Check sheet for the drawn part. Datum: minimum x, y, z corner. Units: mm. Give positions to 0.01 mm unless a question says otherwise; leave off trailing zeros. Order: outer loops, then holes, each group sorted by start corner. A loop starts at its lowest first (then second) coordinate and runs counter-clockwise, first axis right, second up.
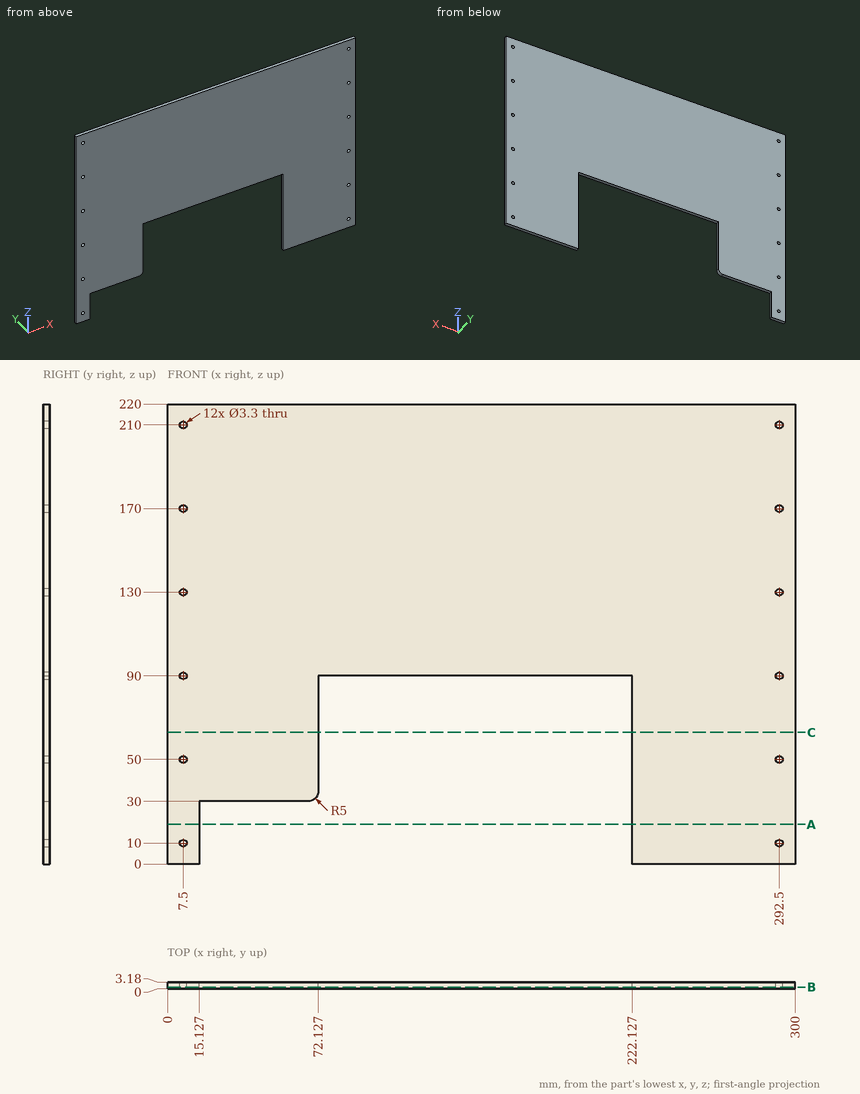
(1) Section check C-C, the plane z = 63. Enter the section's corners in (x, y).
Solved:
outline: (0, 0) - (72.13, 0) - (72.13, 3.18) - (0, 3.18) - close; (222.13, 0) - (300, 0) - (300, 3.18) - (222.13, 3.18) - close
(2) Go/stop test with flat-tipped pins: pin 1 (5.5 mm diameter, centred on x = 7.5, z = 10, fed in from +Y); pin 2 (3 mm diameter, centred on x = 292.5, z = 10, fed in from +Y); pin 3 (1 mm diameter, centred on x = 38.5, y = 1.5, fed in from -Z). Record where each tip stops, or that it passes through.
Solved:
pin 1: stops at y = 3.18
pin 2: passes through
pin 3: stops at z = 30
(3) Scan lines: line 1 (X direction, y = 0.95, z = 170); line 2 (X direction, y = 2.95, z = 44.5); line 3 (X direction, y = 1.8, z = 10). Record each from-to range of solid material in increasing order.
Solved:
line 1: x = 0 to 5.85, 9.15 to 290.85, 294.15 to 300
line 2: x = 0 to 72.13, 222.13 to 300
line 3: x = 0 to 5.85, 9.15 to 15.13, 222.13 to 290.85, 294.15 to 300
(4) Section check A-A, the plane z = 19. Enter the section's corners in (x, y).
Solved:
outline: (0, 0) - (15.13, 0) - (15.13, 3.18) - (0, 3.18) - close; (222.13, 0) - (300, 0) - (300, 3.18) - (222.13, 3.18) - close
(5) Section check B-B, the plane y = 0.75. Give the number of separate pieces and of enclosed holes in the cut face, then the cut area to 3 significant figures.
Solved:
separate pieces: 1
enclosed holes: 12
area: 50,700 mm2
